```python
from build123d import *

# Parameters (mm, degrees)
F1_DEPTH = 25.4
F3_DEPTH = 25.4
F5_DEPTH = 114


# Not quite as in the source:
# - an extrude ends at something that could not be found from the text; its depth is read off the source's solid


with BuildPart() as f1:
    # F0 (on Top) → F1 (new body)
    with BuildSketch(Plane.XY):
        Polygon((-25.4796925148, 25.4), (-25.4796925148, 0), (-46.1431506129, -20.4890353627), (-37.1832725133, -29.489623368), (-19.1820965027, -11.569867169), (-1.2623403036, -29.5710431796), (7.7382477017, -20.61116508), (-12.7796925148, 0), (-12.7796925148, 25.4), align=None)
    extrude(amount=F1_DEPTH)

    # F2 (on face) → F3 (join)
    with BuildSketch(Plane.XY.offset(25.4)):
        with BuildLine():
            Line((-25.4796925148, 25.4), (-12.7796925148, 25.4))
            ThreePointArc((-12.7796925148, 25.4), (-19.1296925148, 31.75), (-25.4796925148, 25.4))
        make_face()
        with BuildLine():
            Line((7.7382477017, -20.61116508), (-1.2623403036, -29.5710431796))
            ThreePointArc((-1.2623403036, -29.5710431796), (7.7178927488, -29.5913981325), (7.7382477017, -20.61116508))
        make_face()
        with BuildLine():
            ThreePointArc((-46.1431506129, -20.4890353627), (-46.1635055657, -29.4692684152), (-37.1832725133, -29.489623368))
            Line((-37.1832725133, -29.489623368), (-46.1431506129, -20.4890353627))
        make_face()
    extrude(amount=-F3_DEPTH)

    # F4 (on face) → F5 (cut, through all)
    with BuildSketch(Plane.XY.offset(25.4)):
        with BuildLine():
            Line((-42.5259842963, -16.9024019821), (-40.6344192228, -15.0268038369))
            ThreePointArc((-40.6344192228, -15.0268038369), (-41.6786510297, -15.8653155428), (-42.5259842963, -16.9024019821))
        make_face()
        with BuildLine():
            ThreePointArc((-32.6380296989, -24.9649388112), (-31.2402342157, -22.88066907), (-30.7492439593, -20.4195837129))
            ThreePointArc((-30.7492439593, -20.4195837129), (-34.0912883888, -14.7893358325), (-40.6344192228, -15.0268038369))
            Line((-40.6344192228, -15.0268038369), (-42.5259842963, -16.9024019821))
            ThreePointArc((-42.5259842963, -16.9024019821), (-41.2158295319, -25.3902171382), (-32.6380296989, -24.9649388112))
        make_face()
        with BuildLine():
            ThreePointArc((3.3359301315, -18.6069775374), (2.8926555851, -16.371867323), (1.6299325028, -14.4750962741))
            ThreePointArc((1.6299325028, -14.4750962741), (-7.9341003982, -20.8420877519), (3.3359301315, -18.6069775374))
        make_face()
    extrude(amount=F5_DEPTH, mode=Mode.SUBTRACT)


solid = f1.part
```
Check sheet for the modelled part. Datum: model origin and axes. Units: mm. A direction names the side the tool comes from. Give positions to 0.01 mm unless a question says otherwise; leave off trailing zeros. Loops run counter-clockwise (first coordinate to the right, second up) from the corner with the lowest first, then second, coordinate; pieces in that order, holes last. Notation, with made-up numbers: M 57,83 L 89,83 A13 cw 89,95 Z; hole C 14.5,88.5 d11. An arc over 180 degrees is marked long. Answer as CSV lines item,"result".
Item 1: Depth check by flat-ended pin: pin 1 Ø12.5 at (y, z) = (10.5, 12) entering from -X; pin 2 Ø1.5 at (x, z) = (-24.5, 15.5) entering from -Y; pin 3 Ø2 at (x, z) = (-9, 2.5) entering from -Y. Enter the tip coordinate at first touch or a pass-through.
Reply:
pin 1,"x = -25.48"
pin 2,"y = -17.61"
pin 3,"y = -22.8"
Item 2: Draft check along X on faces 1 (the face through (-19, -7, 25.4)), 2 (the face through (-10.35, -20.44, 12.52)), 3 (the face through (-25.48, 13, 13)). Enter one of: pulls with the +X half, pulls with the -X half, needs draft (parallel to the pull), parting line crosses it, or undercut.
Reply:
face 1,"needs draft"
face 2,"undercut"
face 3,"pulls with the -X half"
Item 3: Sectioned sample at B-B, the plane y = -5. Enter the section's corners in (x, z), then the cut area to 3 significant figures.
Reply:
outline,"M -30.52,0 L -7.8,0 L -7.8,25.4 L -30.52,25.4 Z"
area,"577 mm^2"
Item 4: Set-up check for faces 4 (the face through (-28.309, -20.655, 12.522)), 5 (the face through (-46.26, -29.37, 12.88)), 6 (the face through (-12.78, 13, 13)): record each of +Z, -Z, +X, -X, +Y, -Y from which the full face is reachable in a straight line by a thin tool's end or side.
Reply:
face 4,"+Z, -Z, -Y"
face 5,"+Z, -Z"
face 6,"+Z, -Z, +X, +Y"
Item 5: Sectioned sample at C-C, the plane x = 3. Enter the section's corners in (y, z), then the cut area to 3 significant figures.
Reply:
outline,"M -31.44,0 L -15.85,0 L -15.85,25.4 L -31.44,25.4 Z"
area,"396 mm^2"
Item 6: Sectioned sample at A-A, the plane z = 5.75. Enter the section's corners in (x, y).
Reply:
outline,"M -46.14,-20.49 A6.35 ccw -37.18,-29.49 L -19.18,-11.57 L -1.26,-29.57 A6.35 ccw 7.74,-20.61 L -12.78,0 L -12.78,25.4 A6.35 ccw -25.48,25.4 L -25.48,0 Z"
Item 7: Scan lines: L1, parallel to X at y = 3, z = 20.25; L2, parallel to X at y = -19, z = 4; L3, parallel to X at y = -23, z = 21.25. Record each from-to range of solid material in increasing order.
Reply:
L1,"-25.48 to -12.78"
L2,"-44.64 to -26.65, -11.79 to 6.13"
L3,"-47.69 to -30.66, -7.8 to 9.23"
